Here's how the part is built. I have some questions about the finished solid (model axes, mm). A direction names the side the tool comes from. Coordinates: 2 decimals unless noted, no trailing zeros. Write each loop counter-clockwise with the first axis right and the second up, starting at its lowest first coordinate (ties: lowest second). Pieces come first, ordered by that corner, then holes. Notation, with made-up numbers: (43, 14.25) - (60, 14.25) arc R21 cw to (60, 21.25) - close; hole circle Ø10 at (57.5, 61). An arc over 180 degrees is marked (long way). Answer in a Markdown table with one row per item. Add a question column.
Item 1: Which directions (+Z, -Z, +X, -X, +Y, -Y) give clear straight access to the entire face, cutting with the end or side of a thin tool? Please do faces 4 (the face through (0, -31, 17)), 5 (the face through (6, -30, 0)).
Item 2: If I drill on probe 1 along Y at (x, z) = (7, 6); probe 2 along Z at (x, y) = (3.5, -38.5); probe 3 along X at (y, z) = (-17.5, 20), over which ranges is the centre line in solid material (lowest first)? Write a range as from..to.
Item 3: Imagine slicing it at A-A (y = -55). Please give me the cut outline in (x, z).
Item 4: We'd pull the mould along Y, two halves only. Please class faces 1 (the face through (5, -62.2, 13)), 2 (the face through (5, -31, -2)), 3 (the face through (6, 0, 13)): +Y half, -Y half, draft (parallel to the pull), parting line (faces both ways), or undercut.
Item 5: Imagine slicing it at C-C (x = 8.25). Please give me the cut outline in (y, z), plus the area to 3 significant figures.
Item 6: I'm going to push a flat-ended pin straight in: pin 1 (4 mm diameter, centred on y = -52.5, z = 11, fed in from +X). Where does the tip first touch, or does it pass through?
Item 7: Imagine slicing it at B-B (z = 24). Please give me the cut outline in (x, y), plus the area to 3 significant figures.
from build123d import *

# Parameters (mm, degrees)
F1_DEPTH = 2
F2_DEPTH = 10


with BuildPart() as f1:
    # F0 (on Right) → F1 (new body)
    with BuildSketch(Plane.YZ):
        Polygon((2, 0), (0, 0), (-30.1, 0), (-60.2, 0), (-62.2, 0), (-62.2, -2), (2, -2), align=None)
        Polygon((0, 26.2), (0, 0), (2, 0), (2, 28.2), (-30.1, 28.2), (-30.1, 26.2), align=None)
        with BuildLine():
            Line((-60.2, 0), (-30.1, 0))
            Line((-30.1, 0), (-30.1, 11.6))
            ThreePointArc((-30.1, 11.6), (-31.16066, 12.03934), (-31.6, 13.1))
            ThreePointArc((-31.6, 13.1), (-31.16066, 14.16066), (-30.1, 14.6))
            Line((-30.1, 14.6), (-30.1, 26.2))
            Line((-30.1, 26.2), (-60.2, 26.2))
            Line((-60.2, 26.2), (-60.2, 0))
        make_face()
        Polygon((-62.2, 0), (-60.2, 0), (-60.2, 26.2), (-30.1, 26.2), (-30.1, 28.2), (-62.2, 28.2), align=None)
        with BuildLine():
            Line((-30.1, 0), (0, 0))
            Line((0, 0), (0, 26.2))
            Line((0, 26.2), (-30.1, 26.2))
            Line((-30.1, 26.2), (-30.1, 14.6))
            ThreePointArc((-30.1, 14.6), (-29.03934, 14.16066), (-28.6, 13.1))
            ThreePointArc((-28.6, 13.1), (-29.03934, 12.03934), (-30.1, 11.6))
            Line((-30.1, 11.6), (-30.1, 0))
        make_face()
    extrude(amount=F1_DEPTH)

    # F0 (on Right) → F2 (join)
    with BuildSketch(Plane.YZ):
        Polygon((0, 26.2), (0, 0), (2, 0), (2, 28.2), (-30.1, 28.2), (-30.1, 26.2), align=None)
        Polygon((2, 0), (0, 0), (-30.1, 0), (-60.2, 0), (-62.2, 0), (-62.2, -2), (2, -2), align=None)
        Polygon((-62.2, 0), (-60.2, 0), (-60.2, 26.2), (-30.1, 26.2), (-30.1, 28.2), (-62.2, 28.2), align=None)
    extrude(amount=F2_DEPTH)


solid = f1.part
Here are the results:
| question | item | result |
|---|---|---|
| 1 | face 4 | +Z, -Z, -X, +Y, -Y |
| 1 | face 5 | +X |
| 2 | probe 1 | y = -62.2..-60.2, 0..2 |
| 2 | probe 2 | z = -2..0, 26.2..28.2 |
| 2 | probe 3 | x = 0..2 |
| 3 | outline | (0, -2) - (10, -2) - (10, 0) - (2, 0) - (2, 26.2) - (10, 26.2) - (10, 28.2) - (0, 28.2) - close |
| 4 | face 1 | -Y half |
| 4 | face 2 | draft |
| 4 | face 3 | undercut |
| 5 | outline | (-62.2, -2) - (2, -2) - (2, 28.2) - (-62.2, 28.2) - close; hole (-60.2, 0) - (0, 0) - (0, 26.2) - (-60.2, 26.2) - close |
| 5 | area | 362 mm2 |
| 6 | pin 1 | stops at x = 2 |
| 7 | outline | (0, -62.2) - (10, -62.2) - (10, -60.2) - (2, -60.2) - (2, 0) - (10, 0) - (10, 2) - (0, 2) - close |
| 7 | area | 160 mm2 |
